Geometry check sheet. Reference: the model listing, model coordinates, mm. Round coordinates to 2 decimals unless told otherwise and drop trailing zeros. Use one line per item in the form item = value.
from build123d import *

# Parameters (mm, degrees)
F0_R     = 5.125
F2_DEPTH = 10
F1_W     = 2
F1_H     = 2.2
F1_W_2   = 2.2
F3_DEPTH = 10


with BuildPart() as f2:
    # F0 (on Top) → F2 (new body)
    with BuildSketch(Plane.XY):
        with BuildLine():
            ThreePointArc((61.8, 59.8), (61.214214, 61.214214), (59.8, 61.8))
            Line((59.8, 61.8), (-59.8, 61.8))
            ThreePointArc((-59.8, 61.8), (-61.214214, 61.214214), (-61.8, 59.8))
            Line((-61.8, 59.8), (-61.8, -59.8))
            ThreePointArc((-61.8, -59.8), (-61.214214, -61.214214), (-59.8, -61.8))
            Line((-59.8, -61.8), (59.8, -61.8))
            ThreePointArc((59.8, -61.8), (61.214214, -61.214214), (61.8, -59.8))
            Line((61.8, -59.8), (61.8, 59.8))
        make_face()
        with Locations((-54, -54)):
            Circle(F0_R, mode=Mode.SUBTRACT)
        with Locations((-40.5, -54)):
            Circle(F0_R, mode=Mode.SUBTRACT)
        with Locations((-54, -40.5)):
            Circle(F0_R, mode=Mode.SUBTRACT)
        with Locations((-40.5, -40.5)):
            Circle(F0_R, mode=Mode.SUBTRACT)
        with Locations((-27, -54)):
            Circle(F0_R, mode=Mode.SUBTRACT)
        with Locations((-13.5, -54)):
            Circle(F0_R, mode=Mode.SUBTRACT)
        with Locations((-27, -40.5)):
            Circle(F0_R, mode=Mode.SUBTRACT)
        with Locations((-13.5, -40.5)):
            Circle(F0_R, mode=Mode.SUBTRACT)
        with Locations((-54, -27)):
            Circle(F0_R, mode=Mode.SUBTRACT)
        with Locations((-40.5, -27)):
            Circle(F0_R, mode=Mode.SUBTRACT)
        with Locations((-54, -13.5)):
            Circle(F0_R, mode=Mode.SUBTRACT)
        with Locations((-40.5, -13.5)):
            Circle(F0_R, mode=Mode.SUBTRACT)
        with Locations((-27, -27)):
            Circle(F0_R, mode=Mode.SUBTRACT)
        with Locations((-13.5, -27)):
            Circle(F0_R, mode=Mode.SUBTRACT)
        with Locations((-27, -13.5)):
            Circle(F0_R, mode=Mode.SUBTRACT)
        with Locations((-13.5, -13.5)):
            Circle(F0_R, mode=Mode.SUBTRACT)
        with Locations((0, -54)):
            Circle(F0_R, mode=Mode.SUBTRACT)
        with Locations((13.5, -54)):
            Circle(F0_R, mode=Mode.SUBTRACT)
        with Locations((27, -54)):
            Circle(F0_R, mode=Mode.SUBTRACT)
        with Locations((0, -40.5)):
            Circle(F0_R, mode=Mode.SUBTRACT)
        with Locations((13.5, -40.5)):
            Circle(F0_R, mode=Mode.SUBTRACT)
        with Locations((27, -40.5)):
            Circle(F0_R, mode=Mode.SUBTRACT)
        with Locations((40.5, -54)):
            Circle(F0_R, mode=Mode.SUBTRACT)
        with Locations((54, -54)):
            Circle(F0_R, mode=Mode.SUBTRACT)
        with Locations((40.5, -40.5)):
            Circle(F0_R, mode=Mode.SUBTRACT)
        with Locations((54, -40.5)):
            Circle(F0_R, mode=Mode.SUBTRACT)
        with Locations((0, -27)):
            Circle(F0_R, mode=Mode.SUBTRACT)
        with Locations((13.5, -27)):
            Circle(F0_R, mode=Mode.SUBTRACT)
        with Locations((27, -27)):
            Circle(F0_R, mode=Mode.SUBTRACT)
        with Locations((0, -13.5)):
            Circle(F0_R, mode=Mode.SUBTRACT)
        with Locations((13.5, -13.5)):
            Circle(F0_R, mode=Mode.SUBTRACT)
        with Locations((27, -13.5)):
            Circle(F0_R, mode=Mode.SUBTRACT)
        with Locations((40.5, -27)):
            Circle(F0_R, mode=Mode.SUBTRACT)
        with Locations((54, -27)):
            Circle(F0_R, mode=Mode.SUBTRACT)
        with Locations((40.5, -13.5)):
            Circle(F0_R, mode=Mode.SUBTRACT)
        with Locations((54, -13.5)):
            Circle(F0_R, mode=Mode.SUBTRACT)
        with Locations((-54, 0)):
            Circle(F0_R, mode=Mode.SUBTRACT)
        with Locations((-54, 13.5)):
            Circle(F0_R, mode=Mode.SUBTRACT)
        with Locations((-40.5, 0)):
            Circle(F0_R, mode=Mode.SUBTRACT)
        with Locations((-40.5, 13.5)):
            Circle(F0_R, mode=Mode.SUBTRACT)
        with Locations((-54, 27)):
            Circle(F0_R, mode=Mode.SUBTRACT)
        with Locations((-40.5, 27)):
            Circle(F0_R, mode=Mode.SUBTRACT)
        with Locations((-27, 0)):
            Circle(F0_R, mode=Mode.SUBTRACT)
        with Locations((-27, 13.5)):
            Circle(F0_R, mode=Mode.SUBTRACT)
        with Locations((-13.5, 0)):
            Circle(F0_R, mode=Mode.SUBTRACT)
        with Locations((-13.5, 13.5)):
            Circle(F0_R, mode=Mode.SUBTRACT)
        with Locations((-27, 27)):
            Circle(F0_R, mode=Mode.SUBTRACT)
        with Locations((-13.5, 27)):
            Circle(F0_R, mode=Mode.SUBTRACT)
        with Locations((-54, 40.5)):
            Circle(F0_R, mode=Mode.SUBTRACT)
        with Locations((-40.5, 40.5)):
            Circle(F0_R, mode=Mode.SUBTRACT)
        with Locations((-54, 54)):
            Circle(F0_R, mode=Mode.SUBTRACT)
        with Locations((-40.5, 54)):
            Circle(F0_R, mode=Mode.SUBTRACT)
        with Locations((-27, 40.5)):
            Circle(F0_R, mode=Mode.SUBTRACT)
        with Locations((-13.5, 40.5)):
            Circle(F0_R, mode=Mode.SUBTRACT)
        with Locations((-27, 54)):
            Circle(F0_R, mode=Mode.SUBTRACT)
        with Locations((-13.5, 54)):
            Circle(F0_R, mode=Mode.SUBTRACT)
        Circle(F0_R, mode=Mode.SUBTRACT)
        with Locations((13.5, 0)):
            Circle(F0_R, mode=Mode.SUBTRACT)
        with Locations((0, 13.5)):
            Circle(F0_R, mode=Mode.SUBTRACT)
        with Locations((13.5, 13.5)):
            Circle(F0_R, mode=Mode.SUBTRACT)
        with Locations((27, 0)):
            Circle(F0_R, mode=Mode.SUBTRACT)
        with Locations((27, 13.5)):
            Circle(F0_R, mode=Mode.SUBTRACT)
        with Locations((0, 27)):
            Circle(F0_R, mode=Mode.SUBTRACT)
        with Locations((13.5, 27)):
            Circle(F0_R, mode=Mode.SUBTRACT)
        with Locations((27, 27)):
            Circle(F0_R, mode=Mode.SUBTRACT)
        with Locations((40.5, 0)):
            Circle(F0_R, mode=Mode.SUBTRACT)
        with Locations((40.5, 13.5)):
            Circle(F0_R, mode=Mode.SUBTRACT)
        with Locations((54, 0)):
            Circle(F0_R, mode=Mode.SUBTRACT)
        with Locations((54, 13.5)):
            Circle(F0_R, mode=Mode.SUBTRACT)
        with Locations((40.5, 27)):
            Circle(F0_R, mode=Mode.SUBTRACT)
        with Locations((54, 27)):
            Circle(F0_R, mode=Mode.SUBTRACT)
        with Locations((0, 40.5)):
            Circle(F0_R, mode=Mode.SUBTRACT)
        with Locations((13.5, 40.5)):
            Circle(F0_R, mode=Mode.SUBTRACT)
        with Locations((27, 40.5)):
            Circle(F0_R, mode=Mode.SUBTRACT)
        with Locations((0, 54)):
            Circle(F0_R, mode=Mode.SUBTRACT)
        with Locations((13.5, 54)):
            Circle(F0_R, mode=Mode.SUBTRACT)
        with Locations((27, 54)):
            Circle(F0_R, mode=Mode.SUBTRACT)
        with Locations((40.5, 40.5)):
            Circle(F0_R, mode=Mode.SUBTRACT)
        with Locations((54, 40.5)):
            Circle(F0_R, mode=Mode.SUBTRACT)
        with Locations((40.5, 54)):
            Circle(F0_R, mode=Mode.SUBTRACT)
        with Locations((54, 54)):
            Circle(F0_R, mode=Mode.SUBTRACT)
    extrude(amount=F2_DEPTH)

    # F1 (on Top) → F3 (cut)
    with BuildSketch(Plane.XY):
        with Locations((-34.3, 61.8)):
            Rectangle(F1_W, F1_H)
        with Locations((34.3, 61.8)):
            Rectangle(F1_W_2, F1_H)
        with Locations((61.8, 34.3)):
            Rectangle(F1_W_2, F1_H)
        with Locations((61.8, -34.3)):
            Rectangle(F1_W_2, F1_H)
        with Locations((34.3, -61.8)):
            Rectangle(F1_W, F1_H)
        with Locations((-34.3, -61.8)):
            Rectangle(F1_W, F1_H)
        with Locations((-61.8, -34.3)):
            Rectangle(F1_W, F1_H)
        with Locations((-61.8, 34.3)):
            Rectangle(F1_W, F1_H)
    extrude(amount=F3_DEPTH, mode=Mode.SUBTRACT)


solid = f2.part
1. Material ranges on line 1 along Y through (x, z) = (35, 8.5), recorded low to high.
Return value:
line_1 = -60.7 to 60.7
2. Gauge pin test, flat ends, axial feed: pin 1 (0.6 mm diameter, centred on x = 61, z = 5, fed in from +Y); pin 2 (1.2 mm diameter, centred on y = 61, z = 5, fed in from -X); pin 3 (0.8 mm diameter, centred on x = -61.5, z = 6, fed in from -Y). Record the tip position at first contact, or that the pin passes through.
Return value:
pin_1 = 61.59
pin_2 = -61.71
pin_3 = -61.32
3. Mould release check, pull along Y, two halves, no side actions. Record for faces 1 (the flat face through (61.8, -48, 5)), 2 (the cylindrical face through (56.36, 22.45, 4.93)): released by +Y, released by -Y, zero draft, split by the parting line, or undercut.
Return value:
face_1 = zero draft
face_2 = undercut
4. Section check A-A (y = -13.5). Count the separate pieces of the cut face and the enclosed holes in it, then the cut area to 4 significant figures.
Return value:
separate_pieces = 10
enclosed_holes = 0
area = 313.5 mm2
